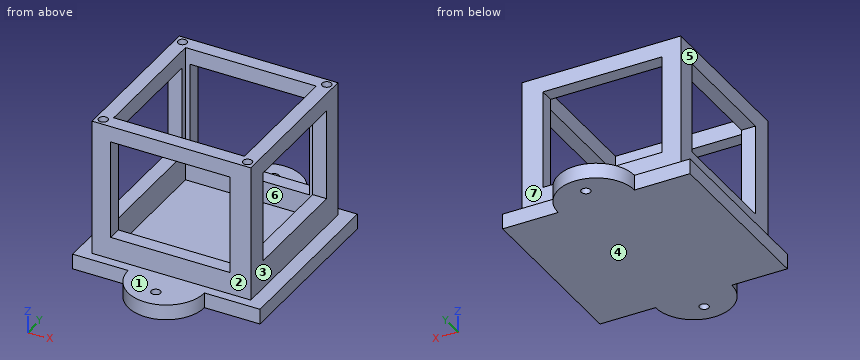
Autodesk Inventor part; units mm, degrees
ref_plane "YZ Plane" through (0, 0, 0) normal (1, 0, 0) x (0, 1, 0)
ref_plane "XZ Plane" through (0, 0, 0) normal (0, 1, 0) x (-1, 0, 0)
ref_plane "XY Plane" through (0, 0, 0) normal (0, 0, 1) x (1, 0, 0)
sketch "Boceto1" plane through (0, 0, 0) normal (0, 0, 1) x (1, 0, 0)
  line L0 (-26, -26) -> (26, -26)
  line L1 (26, -26) -> (26, 26)
  line L2 (26, 26) -> (-26, 26)
  line L3 (-26, 26) -> (-26, -26)
  line L4 (-26, -26) -> (26, 26) construction
  line L5 (26, -26) -> (-26, 26) construction
  circle A0 centre (-23.6478, 23.6478) radius 1.5
  circle A1 centre (23.6478, 23.6478) radius 1.5
  circle A2 centre (23.6478, -23.6478) radius 1.5
  line L6 (-21.4311, -21.4311) -> (21.4311, -21.4311)
  line L7 (21.4311, -21.4311) -> (21.4311, 21.4311)
  line L8 (21.4311, 21.4311) -> (-21.4311, 21.4311)
  line L9 (-21.4311, 21.4311) -> (-21.4311, -21.4311)
  line L10 (-21.4311, -21.4311) -> (21.4311, 21.4311) construction
  line L11 (21.4311, -21.4311) -> (-21.4311, 21.4311) construction
  circle A3 centre (-23.6478, -23.6478) radius 1.5
  point P0 (0, 0)
  dimension "d0" = 52
  dimension "d1" = 52
  dimension "d2" = 3
  dimension "d3" = 3
  dimension "d4" = 3
  dimension "d6" = 3
extrude "Extrusión1" add sketch "Boceto1" along normal blind 45
sketch "Boceto2" plane through (0, 0, 0) normal (0, 0, -1) x (-1, 0, 0)
  line L0 (30.6977, 29.0649) -> (-30.6977, 29.0649)
  line L1 (-30.6977, 29.0649) -> (-30.6977, -29.0649)
  line L2 (-30.6977, -29.0649) -> (30.6977, -29.0649)
  line L3 (30.6977, -29.0649) -> (30.6977, 29.0649)
  line L4 (30.6977, 29.0649) -> (-30.6977, -29.0649) construction
  line L5 (-30.6977, 29.0649) -> (30.6977, -29.0649) construction
  point P0 (0, 0)
extrude "Extrusión2" add sketch "Boceto2" along normal blind 5
thread "Rosca1"
thread "Rosca2"
thread "Rosca3"
thread "Rosca4"
sketch "Boceto3" plane through (0, 0, -5) normal (0, 0, -1) x (-1, 0, 0)
  line L0 (-30.6977, -29.0649) -> (30.6977, -29.0649)
  arc A0 (-12.5, -29.0649) -> (12.5, -29.0649) centre (0, -29.0649) ccw
  line L1 (30.6977, 29.0649) -> (-30.6977, 29.0649)
  arc A1 (12.5, 29.0649) -> (-12.5, 29.0649) centre (0, 29.0649) ccw
  circle A2 centre (0, -35.3149) radius 1.5
  circle A3 centre (0, 35.3149) radius 1.5
  point P0 (0, 0)
  dimension "d19" = 25
  dimension "d20" = 25
  dimension "d21" = 3
  dimension "d22" = 3
extrude "Extrusión3" add sketch "Boceto3" against normal blind 5
thread "Rosca5"
thread "Rosca6"
sketch "Boceto4" plane through (26, -26, 45) normal (1, 0, 0) x (0, 0, -1)
  line L0 (5.7927, 7.3891) -> (35.7255, 7.3891)
  line L1 (35.7255, 7.3891) -> (35.7255, 45.2774)
  line L2 (35.7255, 45.2774) -> (5.7927, 45.2774)
  line L3 (5.7927, 45.2774) -> (5.7927, 7.3891)
  point P0 (45, 26)
extrude "Extrusión4" cut sketch "Boceto4" against normal blind 66
sketch "Boceto5" plane through (-26, 26, 45) normal (0, 1, 0) x (1, 0, 0)
  line L0 (45.1937, 5.2117) -> (6.1058, 5.2117)
  line L1 (6.1058, 5.2117) -> (6.1058, 37.7148)
  line L2 (6.1058, 37.7148) -> (45.1937, 37.7148)
  line L3 (45.1937, 37.7148) -> (45.1937, 5.2117)
  point P0 (26, 45)
extrude "Extrusión5" cut sketch "Boceto5" against normal blind 66
properties part number "Base para Driver Corregida"
Could you check a few things on this model? Use its own coordinates, in mm. Face numbers are marked on the shaded views. A direction names the side the tool comes from. Round coordinates to 2 decimals unless told otherwise and drop trailing zeros. Loops run counter-clockwise (first coordinate to the right, second up) from the corner with the lowest first, then second, coordinate; pieces in that order, holes last. Notation, with made-up numbers: M -17,-20.75 L 18,-20.75 A18 ccw 18,-6.75 Z; hole C -9.5,51 d10. An arc over 180 degrees is marked long. Write item = value, one per line.
1. I need wall thicknesses on probe 1 along Y at (x, z) = (0, -1.7); probe 2 along Z at (x, y) = (-25.5, -11); probe 3 along X at (y, z) = (-14.5, 2.5). Which ranges of each line are inside material? Lowest first, please.
Results below:
probe_1 = -41.56 to -36.81, -33.81 to 33.81, 36.81 to 41.56
probe_2 = -5 to 9.27, 39.21 to 45
probe_3 = -26 to -21.43, 21.43 to 26
2. I want a section at D-D, the plane x = 0. Write out the boundary of the cut face in (y, z).
Results below:
outline = M -41.56,-5 L -36.81,-5 L -36.81,0 L -41.56,0 Z; M -33.81,-5 L 33.81,-5 L 33.81,0 L 26,0 L 26,7.29 L 21.43,7.29 L 21.43,0 L -21.43,0 L -21.43,7.29 L -26,7.29 L -26,0 L -33.81,0 Z; M -26,39.79 L -21.43,39.79 L -21.43,45 L -26,45 Z; M 21.43,39.79 L 26,39.79 L 26,45 L 21.43,45 Z; M 36.81,-5 L 41.56,-5 L 41.56,0 L 36.81,0 Z
3. Thinking about a two-plate mould opening in X: for the marked faces 5, 6 and 7, which applies, +X half, -X half, draft (parallel to the pull), parting line (faces both ways), or undercut?
Results below:
face_5 = -X half
face_6 = undercut
face_7 = draft
4. Will these pins go through, and if not, where does the flat tip stop? P1, Ø21.5, axis at y = -6.5, z = 19, coming from the +X side; P2, Ø5.5, axis at x = -20.5, z = -2, coming from the -Y side; P3, Ø10, axis at y = -10, z = 29.5, coming from the -X side; P4, Ø1.5, axis at x = -21.5, z = -1.5, coming from the +Y side.
Results below:
P1 = 26
P2 = -29.06
P3 = through
P4 = 29.06
5. I want a section at A-A, the plane x = 16.5. Write out the boundary of the cut face in (y, z).
Results below:
outline = M -29.06,-5 L 29.06,-5 L 29.06,0 L 26,0 L 26,7.29 L 21.43,7.29 L 21.43,0 L -21.43,0 L -21.43,7.29 L -26,7.29 L -26,0 L -29.06,0 Z; M -26,39.79 L -21.43,39.79 L -21.43,45 L -26,45 Z; M 21.43,39.79 L 26,39.79 L 26,45 L 21.43,45 Z
6. I want a section at C-C, the plane y = -17.5. Write out the boundary of the cut face in (x, z), and give its area (3 significant figures).
Results below:
outline = M -30.7,-5 L 30.7,-5 L 30.7,0 L 26,0 L 26,9.27 L 21.43,9.27 L 21.43,0 L -21.43,0 L -21.43,9.27 L -26,9.27 L -26,0 L -30.7,0 Z; M -26,39.21 L -21.43,39.21 L -21.43,45 L -26,45 Z; M 21.43,39.21 L 26,39.21 L 26,45 L 21.43,45 Z
area = 445 mm²
7. I want a section at B-B, the plane z = 36. Write out the boundary of the cut face in (x, y), and give its area (3 significant figures).
Results below:
outline = M -26,-26 L -19.89,-26 L -19.89,-21.43 L -21.43,-21.43 L -21.43,-18.61 L -26,-18.61 Z; M -26,19.28 L -21.43,19.28 L -21.43,21.43 L -19.89,21.43 L -19.89,26 L -26,26 Z; M 19.19,-26 L 26,-26 L 26,-18.61 L 21.43,-18.61 L 21.43,-21.43 L 19.19,-21.43 Z; M 19.19,21.43 L 21.43,21.43 L 21.43,19.28 L 26,19.28 L 26,26 L 19.19,26 Z; hole C -23.65,-23.65 d3; hole C -23.65,23.65 d3; hole C 23.65,-23.65 d3; hole C 23.65,23.65 d3
area = 135 mm²
8. Which directions (+Z, -Z, +X, -X, +Y, -Y) give clear straight access to the entire face, cutting with the end or side of a thin tool? Please do the marked faces 1, 2, 3 and 4.
Results below:
face_1 = +Z
face_2 = +Z, +X, -X, -Y
face_3 = +Z, +X, +Y, -Y
face_4 = -Z, +X, -X, +Y, -Y
